```python
from build123d import *

# Parameters (mm, degrees)
SKETCH_R     = 12
SKETCH_R_2   = 21
SKETCH_R_3   = 19.584537
PAD_DEPTH    = 30
PAD001_DEPTH = 30


with BuildPart() as part:
    # Sketch → Pad (new body)
    with BuildSketch(Plane.XY):
        with BuildLine():
            Line((-35.584206, -63.111127), (44.415794, -63.111127))
            ThreePointArc((44.415794, -63.111127), (77.13309, -49.55918), (90.685038, -16.841884))
            Line((90.685038, -16.841884), (90.685038, 63.158116))
            ThreePointArc((90.685038, 63.158116), (77.13309, 95.875412), (44.415794, 109.427359))
            Line((44.415794, 109.427359), (-35.584206, 109.427359))
            ThreePointArc((-35.584206, 109.427359), (-68.301501, 95.875412), (-81.853449, 63.158116))
            Line((-81.853449, 63.158116), (-81.853449, -16.841884))
            ThreePointArc((-81.853449, -16.841884), (-68.301501, -49.55918), (-35.584206, -63.111127))
        make_face()
        with Locations((4.62833, 30.241158)):
            Circle(SKETCH_R, mode=Mode.SUBTRACT)
        with Locations((-50.106209, -31.898642)):
            Circle(SKETCH_R_2, mode=Mode.SUBTRACT)
        with Locations((59.362869, 78.858307)):
            Circle(SKETCH_R_3, mode=Mode.SUBTRACT)
    extrude(amount=PAD_DEPTH)

    # Sketch → Pad001 (join)
    with BuildSketch(Plane.XY):
        with BuildLine():
            Line((-35.584206, -63.111127), (44.415794, -63.111127))
            ThreePointArc((44.415794, -63.111127), (77.13309, -49.55918), (90.685038, -16.841884))
            Line((90.685038, -16.841884), (90.685038, 63.158116))
            ThreePointArc((90.685038, 63.158116), (77.13309, 95.875412), (44.415794, 109.427359))
            Line((44.415794, 109.427359), (-35.584206, 109.427359))
            ThreePointArc((-35.584206, 109.427359), (-68.301501, 95.875412), (-81.853449, 63.158116))
            Line((-81.853449, 63.158116), (-81.853449, -16.841884))
            ThreePointArc((-81.853449, -16.841884), (-68.301501, -49.55918), (-35.584206, -63.111127))
        make_face()
        with Locations((4.62833, 30.241158)):
            Circle(SKETCH_R, mode=Mode.SUBTRACT)
        with Locations((-50.106209, -31.898642)):
            Circle(SKETCH_R_2, mode=Mode.SUBTRACT)
        with Locations((59.362869, 78.858307)):
            Circle(SKETCH_R_3, mode=Mode.SUBTRACT)
    extrude(amount=PAD001_DEPTH)


solid = part.part
```
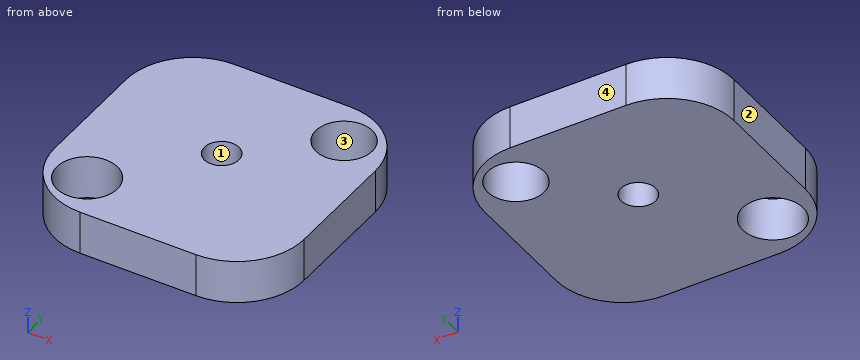
Geometry check sheet. Reference: the model listing, model coordinates, mm. Face numbers are marked on the shaded views. Coordinates: 2 decimals unless noted, no trailing zeros. Order: outer loops, then holes, each group sorted by start corner. A loop starts at its lowest first (then second) coordinate and runs counter-clockwise, first axis right, second up. Notation, with made-up numbers: (11.25, -16.75) - (46.25, -16.75) arc R31 cw to (46.25, 8.25) - close; hole circle Ø1 at (35, 42.5). An arc over 180 degrees is marked (long way). Use one line per item in the form item = value.
1. Section check B-B (y = 74.5). Record the boundary of the cut face in (x, z), then the cut area to 3 significant figures.
Here are the results:
outline = (-80.44, 0) - (40.27, 0) - (40.27, 30) - (-80.44, 30) - close; (78.46, 0) - (89.27, 0) - (89.27, 30) - (78.46, 30) - close
area = 3,950 mm²
2. Scan lines: line 1 (Y direction, x = 4, z = 22.5); line 2 (X direction, y = -14, z = 19); line 3 (X direction, y = 67, z = 17.25). Record each from-to range of solid material in increasing order.
Here are the results:
line_1 = -63.11 to 18.26, 42.22 to 109.43
line_2 = -81.85 to -61.09, -39.12 to 90.69
line_3 = -81.69 to 43.78, 74.95 to 90.53
3. Draft check along X on the marked faces 1, 2, 3 and 4. Enter one of: pulls with the +X half, pulls with the -X half, needs draft (parallel to the pull), parting line crosses it, or undercut.
Here are the results:
face_1 = undercut
face_2 = pulls with the -X half
face_3 = undercut
face_4 = needs draft
4. Section check C-C (z = 24). Record the boundary of the cut face in (x, y).
Here are the results:
outline = (-81.85, -16.84) arc R46.27 ccw to (-35.58, -63.11) - (44.42, -63.11) arc R46.27 ccw to (90.69, -16.84) - (90.69, 63.16) arc R46.27 ccw to (44.42, 109.43) - (-35.58, 109.43) arc R46.27 ccw to (-81.85, 63.16) - close; hole circle Ø42 at (-50.11, -31.9); hole circle Ø24 at (4.63, 30.24); hole circle Ø39.17 at (59.36, 78.86)
5. Section check A-A (x = -54.5). Record the boundary of the cut face in (y, z), then the cut area to 3 significant figures.
Here are the results:
outline = (-59.07, 0) - (-52.43, 0) - (-52.43, 30) - (-59.07, 30) - close; (-11.36, 0) - (105.38, 0) - (105.38, 30) - (-11.36, 30) - close
area = 3,700 mm²
6. Gauge pin test, flat ends, axial feed: pin 1 (2 mm diameter, centred on x = 55, z = 12.5, fed in from -Y); pin 2 (1.5 mm diameter, centred on y = -28, z = 24, fed in from -X). Record the tip position at first contact, or that the pin passes through.
Here are the results:
pin_1 = -62.11
pin_2 = -80.67
